Here's how the part is built. I have some questions about the finished solid (model axes, mm). Coordinates: 2 decimals unless noted, no trailing zeros. Loops run counter-clockwise (first coordinate to the right, second up) from the corner with the lowest first, then second, coordinate; pieces in that order, holes last. Notation, with made-up numbers: (80, 9) - (97, 9) arc R15 cw to (97, 36) - close; hole circle Ø6 at (55, 17). An arc over 180 degrees is marked (long way). Use a Markdown table: item, result.
Autodesk Inventor part; units mm, degrees
ref_plane "YZ Plane" through (0, 0, 0) normal (1, 0, 0) x (0, 1, 0)
ref_plane "XZ Plane" through (0, 0, 0) normal (0, 1, 0) x (-1, 0, 0)
ref_plane "XY Plane" through (0, 0, 0) normal (0, 0, 1) x (1, 0, 0)
sketch "Sketch1" plane through (0, 0, 0) normal (0, 1, 0) x (-1, 0, 0)
  point P0 (0, 0)
sketch "Sketch2" plane through (0, 0, 0) normal (0, 1, 0) x (-1, 0, 0)
  circle A0 centre (0.2711, 0.2358) radius 1.75
  point P0 (0, 0)
  dimension "d0" = 3.5
extrude "Extrusion1" add sketch "Sketch2" along normal blind 7.5
sketch "Sketch5" plane through (-0.2711, 7.5, 0.2358) normal (0, 1, 0) x (1, 0, 0)
  circle A0 centre (0, 0) radius 0.25
  point P0 (0.2711, 0.2358)
sketch "Sketch8" plane through (-0.2711, 0, 0.2358) normal (0, -1, 0) x (1, 0, 0)
  circle A0 centre (0, 0) radius 0.25
  point P0 (0.2711, -0.2358)
  dimension "d24" = 0.5
sketch3d "3D Sketch3"
  line L0 (-0.2711, 0, 0.2358) -> (-0.2711, -22.5, 0.2358)
  arc A0 (-0.2711, -22.5, 0.2358) -> (-0.2711, -25, 2.7358) centre (-0.2711, -22.5, 2.7358) ccw
  line L1 (-0.2711, -25, 2.7358) -> (-0.2711, -25, 12.2358)
  dimension "d21" = 25
  dimension "d22" = 12
  dimension "d23" = 2.5
sweep "Sweep1" add profiles "Sketch8" path "3D Sketch3"
sketch3d "3D Sketch5"
  line L0 (-0.2711, 7.5, 0.2358) -> (-0.2711, 30, 0.2358)
  arc A0 (-0.2711, 30, 0.2358) -> (-0.2711, 32.5, 2.7358) centre (-0.2711, 30, 2.7358) ccw
  line L1 (-0.2711, 32.5, 2.7358) -> (-0.2711, 32.5, 12.2358)
  dimension "d27" = 25
  dimension "d28" = 12
  dimension "d29" = 2.5
sweep "Sweep2" add profiles "Sketch5" path "3D Sketch5"
properties part number "Diode" material "Silicon Nitride"
Q1. I want a section at B-B, the plane z = 1.25. Give the number of separate pieces and of enclosed holes in the cut face, then the cut area to 3 significant figures.
Check values:
| item | result |
|---|---|
| separate pieces | 3 |
| enclosed holes | 0 |
| area | 21.9 mm^2 |
Q2. Please list where these lines run through material, in increasing order: L1, parallel to Y at x = -0.45, z = 1; L2, parallel to Z at x = -0.3, y = -4.5; L3, parallel to Y at x = 0.65, z = 0.5. Write a range as from..to.
Check values:
| item | result |
|---|---|
| L1 | -24.53..-24.05, 0..7.5, 31.55..32.03 |
| L2 | -0.01..0.48 |
| L3 | 0..7.5 |
Q3. I want a section at D-D, the plane x = -1.45. Write out the boundary of the cut face in (y, z), then the cut area to 3 significant figures.
Check values:
| item | result |
|---|---|
| outline | (0, -1.06) - (7.5, -1.06) - (7.5, 1.53) - (0, 1.53) - close |
| area | 19.4 mm^2 |
Q4. I want a section at A-A, the plane z = 5.75. Write out the boundary of the cut face in (x, y).
Check values:
| item | result |
|---|---|
| outline | circle Ø0.5 at (-0.27, -25); circle Ø0.5 at (-0.27, 32.5) |
Q5. I want a section at C-C, the plane y = -13. Write out the boundary of the cut face in (x, z), then the cut area to 3 significant figures.
Check values:
| item | result |
|---|---|
| outline | circle Ø0.5 at (-0.27, 0.24) |
| area | 0.196 mm^2 |
Q6. Will these pins go through, and if not, where does the flat tip stop? P1, Ø4, axis at y = 25.5, z = 4, coming from the +X side; P2, Ø1, axis at x = 0, z = 0.5, coming from the +Y side.
Check values:
| item | result |
|---|---|
| P1 | through |
| P2 | y = 32.08 |
